Read the model definition and answer for the solid it produces. Units are mm, in the model's axes. Coordinates: 2 decimals unless noted, no trailing zeros. Loops run counter-clockwise (first coordinate to the right, second up) from the corner with the lowest first, then second, coordinate; pieces in that order, holes last. Notation, with made-up numbers: (67, 42.25) -> (74, 42.25) arc R29 cw to (74, 77.25) -> close; hole circle Ø4 at (-36, 9.5). An arc over 180 degrees is marked (long way). One line per question, with ' | ' between items. Start each with the question number.
```python
from build123d import *

# Parameters (mm, degrees)
F1_DEPTH    = 5.08
F2_T1_DEPTH = 18.1441495789
F2_T3_DEPTH = 18.1441495789
F2_T5_DEPTH = 18.1441495789
F2_T7_DEPTH = 18.1441495789
F2_T9_DEPTH = 10.8131399699


# Not quite as in the source:
# - a fillet or chamfer that OpenCascade refuses, or shapes differently, is made with other operations: its cross-section is extruded or revolved along the edge and cut away or added


with BuildPart() as f1:
    # F0 (on Front) → F1 (new body)
    with BuildSketch(Plane.XZ):
        Polygon((-25.7146830065, 3.5921024484), (-22.1225805581, 0), (-18.5304781096, 3.5921024484), (-18.5304781096, 16.2921024484), (-22.1225805581, 19.8842048969), (-25.7146830065, 16.2921024484), align=None)
    extrude(amount=F1_DEPTH)

    # F2: chamfer of 2.54 on 12 edges, made by hand

    # F2_s2 → F2_t1 (cut)
    with BuildSketch(Plane(origin=(-12.7924159002, 0, 12.7924159002), x_dir=(0, 1, 0), z_dir=(-0.7071067812, 0, 0.7071067812))):
        Polygon((-2.54, 1.5827706089), (-5.08, 4.1227706089), (-5.08, 1.5827706089), align=None)
        Polygon((-2.54, 1.5827706089), (0, 4.1227706089), (0, 1.5827706089), align=None)
    extrude(amount=F2_T1_DEPTH, mode=Mode.SUBTRACT)

    # F2_s4 → F2_t3 (cut)
    with BuildSketch(Plane(origin=(3.4996865482, 0, 3.4996865482), x_dir=(0, 1, 0), z_dir=(-0.7071067812, 0, -0.7071067812))):
        Polygon((-2.54, -29.703282851), (-5.08, -27.163282851), (-5.08, -29.703282851), align=None)
        Polygon((-2.54, -29.703282851), (0, -27.163282851), (0, -29.703282851), align=None)
    extrude(amount=F2_T3_DEPTH, mode=Mode.SUBTRACT)

    # F2_s6 → F2_t5 (cut)
    with BuildSketch(Plane(origin=(-19.2722671063, 0, 19.2722671063), x_dir=(0, 1, 0), z_dir=(0.7071067812, 0, -0.7071067812))):
        Polygon((-2.54, -15.64302673), (-5.08, -13.10302673), (-5.08, -15.64302673), align=None)
        Polygon((-2.54, -15.64302673), (0, -13.10302673), (0, -15.64302673), align=None)
    extrude(amount=F2_T5_DEPTH, mode=Mode.SUBTRACT)

    # F2_s8 → F2_t7 (cut)
    with BuildSketch(Plane(origin=(-15.6801646579, 0, -15.6801646579), x_dir=(0, 1, 0), z_dir=(0.7071067812, 0, 0.7071067812))):
        Polygon((-2.54, 15.64302673), (-5.08, 18.18302673), (-5.08, 15.64302673), align=None)
        Polygon((-2.54, 15.64302673), (0, 18.18302673), (0, 15.64302673), align=None)
    extrude(amount=F2_T7_DEPTH, mode=Mode.SUBTRACT)

    # F2_s10 → F2_t9 (cut)
    with BuildSketch(Plane.XZ.offset(-2.8665699849)):
        Polygon((-19.2744268854, 2.8481536726), (-18.5304781096, 4.6442048969), (-18.5304781096, 3.5921024484), align=None)
        Polygon((-18.5304781096, 15.24), (-19.2744268854, 17.0360512242), (-18.5304781096, 16.2921024484), align=None)
        Polygon((-25.7146830065, 15.24), (-24.9707342307, 17.0360512242), (-25.7146830065, 16.2921024484), align=None)
        Polygon((-25.7146830065, 4.6442048969), (-24.9707342307, 2.8481536726), (-25.7146830065, 3.5921024484), align=None)
    extrude(amount=F2_T9_DEPTH, mode=Mode.SUBTRACT)


solid = f1.part
```
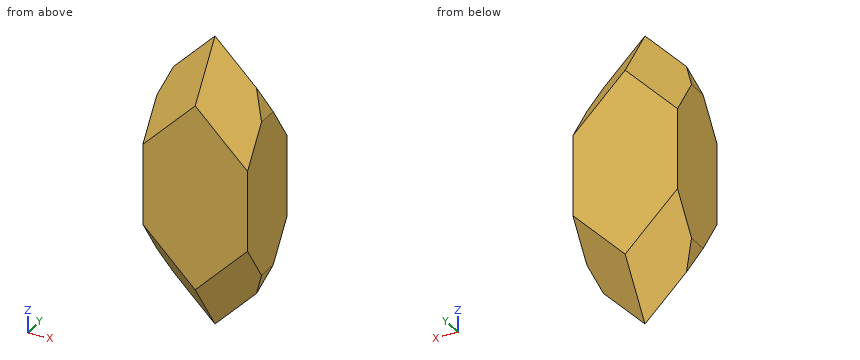
(1) Section D-D on z = 15.75 is taken. Write down the section's boundary in (x, y).
(2) This flat-tipped pin is pushed along its axis until it touches: pin 1 Ø2 at (x, y) = (-24, -3.5) entering from +Z. Where does it stop, or does it pass through?
(3) Section C-C on x = -24 is taken. Write down the section's boundary in (y, z).
(4) Section B-B on y = -1.05 is taken. Write down the section's boundary in (x, z), plus the area to 3 significant figures.
(5) Section A-A on z = 5.25 is taken. Write down the section's boundary in (x, y), plus the area to 3 significant figures.
(6) Find the intervals of material crossed by probe 1 along Z at (x, y) = (-22.25, -1.35); probe 2 along X at (y, z) = (-1.55, 17.5); probe 3 along Z at (x, y) = (-20.25, -0.15), in increasing order. Write a range as from..to.
Working result:
1) outline: (-25.5, -3.07) -> (-22.66, -5.08) -> (-21.58, -5.08) -> (-18.74, -3.07) -> (-18.74, -2.01) -> (-21.58, 0) -> (-22.66, 0) -> (-25.5, -2.01) -> close
2) pin 1: stops at z = 18.38
3) outline: (-5.08, 5.47) -> (-2.54, 1.88) -> (0, 5.47) -> (0, 14.41) -> (-2.54, 18.01) -> (-5.08, 14.41) -> close
4) outline: (-25.71, 5.7) -> (-22.12, 2.11) -> (-18.53, 5.7) -> (-18.53, 14.18) -> (-22.12, 17.78) -> (-25.71, 14.18) -> close | area: 86.8 mm2
5) outline: (-25.71, -3.71) -> (-23.78, -5.08) -> (-20.46, -5.08) -> (-18.53, -3.71) -> (-18.53, -1.37) -> (-20.46, 0) -> (-23.78, 0) -> (-25.71, -1.37) -> close | area: 31.2 mm2
6) probe 1: z = 1.81..18.07 | probe 2: x = -23.11..-21.14 | probe 3: z = 5.25..14.63
